Read the model definition and answer for the solid it produces. Units are mm, in the model's axes. A direction names the side the tool comes from. Give positions to 0.01 mm unless a question says otherwise; leave off trailing zeros. Order: outer loops, then holes, each group sorted by start corner. A loop starts at its lowest first (then second) coordinate and runs counter-clockwise, first axis right, second up. Notation, with made-up numbers: (-3.75, 17) - (17.25, 17) arc R33 ccw to (17.25, 49) - close; hole circle Ø9 at (85.5, -15). An arc over 180 degrees is marked (long way). Write each question's results on one line, items separated by ' | '.
from build123d import *

# Parameters (mm, degrees)
F0_W      = 121
F0_H      = 76
F1_DEPTH  = 6
F2_W      = 121
F2_H      = 78
F3_DEPTH  = 1.6
F4_R      = 1
F5_DEPTH  = 2
F6_W      = 3.5
F6_H      = 9
F7_DEPTH  = 3.5
F8_R      = 1.575
F9_DEPTH  = 16
F10_R     = 1
F11_DEPTH = 19


with BuildPart() as f1:
    # F0 (on Front) → F1 (new body)
    with BuildSketch(Plane.XZ):
        Rectangle(F0_W, F0_H)
    extrude(amount=F1_DEPTH)

    # F2 (on Front) → F3 (join)
    with BuildSketch(Plane.XZ):
        Rectangle(F2_W, F2_H)
    extrude(amount=F3_DEPTH)

    # F4 (on face) → F5 (join)
    with BuildSketch(Plane(origin=(0, 0, 0), x_dir=(-1, 0, 0), z_dir=(0, 1, 0))):
        with Locations((-56.5, 35.5)):
            Circle(F4_R)
        with Locations((-56.5, -34.5)):
            Circle(F4_R)
        with Locations((37, -34.5)):
            Circle(F4_R)
        with Locations((37, 35.5)):
            Circle(F4_R)
    extrude(amount=F5_DEPTH)

    # F6 (on face) → F7 (join)
    with BuildSketch(Plane(origin=(0, 0, 0), x_dir=(-1, 0, 0), z_dir=(0, 1, 0))):
        with Locations((-55.75, -24.5)):
            Rectangle(F6_W, F6_H)
    extrude(amount=F7_DEPTH)

    # F8 (on face) → F9 (join)
    with BuildSketch(Plane(origin=(0, 0, 0), x_dir=(-1, 0, 0), z_dir=(0, 1, 0))):
        with Locations((-56.5, 35.5)):
            Circle(F8_R)
        with Locations((37, 35.5)):
            Circle(F8_R)
        with Locations((-56.5, -34.5)):
            Circle(F8_R)
        with Locations((37, -34.5)):
            Circle(F8_R)
    extrude(amount=F9_DEPTH)

    # F10 (on face) → F11 (join)
    with BuildSketch(Plane(origin=(0, 0, 0), x_dir=(-1, 0, 0), z_dir=(0, 1, 0))):
        with Locations((37, 35.5)):
            Circle(F10_R)
        with Locations((37, -34.5)):
            Circle(F10_R)
        with Locations((-56.5, -34.5)):
            Circle(F10_R)
        with Locations((-56.5, 35.5)):
            Circle(F10_R)
    extrude(amount=F11_DEPTH)


solid = f1.part
(1) Section D-D (y = 17.75) is taken. Give the vertices of the cut face in (x, z), plus the area to 3 significant figures.
Conclusion:
outline: circle Ø2 at (-37, -34.5); circle Ø2 at (-37, 35.5); circle Ø2 at (56.5, -34.5); circle Ø2 at (56.5, 35.5) | area: 12.6 mm^2
(2) Section A-A (z = -26) is taken. Give the vertices of the cut face in (x, y).
Conclusion:
outline: (-60.5, -6) - (60.5, -6) - (60.5, 0) - (57.5, 0) - (57.5, 3.5) - (54, 3.5) - (54, 0) - (-60.5, 0) - close
(3) Consider probe 1 along Y at (x, z) = (-13.5, 25); probe 2 along Z at (x, y) = (32.5, -2.75). Determine where each line is inside the solid, lowest interval first. Write a range as [from, to].
Conclusion:
probe 1: [-6, 0] | probe 2: [-38, 38]
(4) Each of these flat-tipped pins is pushed along its axis until it touches: pin 1 (5 mm diameter, centred on x = -19.5, y = -4.5, fed in from -Z); pin 2 (1.3 mm diameter, centred on x = 28, y = -3, fed in from +Z); pin 3 (3 mm diameter, centred on x = 55.5, z = -24.5, fed in from +Y). Where does it stop, or does it pass through?
Conclusion:
pin 1: z = -38 | pin 2: z = 38 | pin 3: y = 3.5
(5) Section C-C (x = -12) is taken. Give the vertices of the cut face in (y, z).
Conclusion:
outline: (-6, -38) - (-1.6, -38) - (-1.6, -39) - (0, -39) - (0, 39) - (-1.6, 39) - (-1.6, 38) - (-6, 38) - close
(6) Section B-B (y = 9.25) is taken. Give the vertices of the cut face in (x, z) (3 decimals), plus the area to 3 significant figures.
Conclusion:
outline: circle Ø3.15 at (-37, -34.5); circle Ø3.15 at (-37, 35.5); circle Ø3.15 at (56.5, -34.5); circle Ø3.15 at (56.5, 35.5) | area: 31.2 mm^2
(7) The mould has two halves that part along Z. Classify faces 5 (the face through (58.073, 7.888, 35.569)), 6 (the face through (54, 2, -25)), 7 (the face through (-1, -4, 38)): pulls with the +Z half, pulls with the -Z half, needs draft (parallel to the pull), parting line crosses it, or undercut.
Conclusion:
face 5: undercut | face 6: needs draft | face 7: pulls with the +Z half
(8) For faces 1 (the face through (-1, -6, 1)), 2 (the face through (-35.427, 7.888, -34.431)), 3 (the face through (57.5, 2, -25)), 4 (the face through (56, 2, -29)), determine the directions among +Z, -Z, +X, -X, +Y, -Y from which every point of the face is accessible in a straight line to the end or side of a thin tool.
Conclusion:
face 1: +Z, -Z, +X, -X, -Y | face 2: +Y | face 3: +X, +Y | face 4: +X, -X, +Y
